```python
from build123d import *

# Parameters (mm, degrees)
SKETCH1_W           = 2.5
SKETCH1_H           = 2.5
SKETCH1_W_2         = 2
SKETCH1_H_2         = 2
BOSS_EXTRUDE1_DEPTH = 2.5
SCALE1_SCALE        = 6


with BuildPart() as part:
    # Sketch1 → Boss-Extrude1 (new body)
    with BuildSketch(Plane(origin=(0, 0, 0), x_dir=(1, 0, 0), z_dir=(0, 1, 0))):
        Rectangle(SKETCH1_W, SKETCH1_H)
        Rectangle(SKETCH1_W_2, SKETCH1_H_2, mode=Mode.SUBTRACT)
    extrude(amount=BOSS_EXTRUDE1_DEPTH)


with BuildPart() as part_1:
    # Scale1: scaled about (0, 1.25, 0)
    add(part.part.scale(SCALE1_SCALE).moved(Location((0, -6.25, 0))))


solid = part_1.part
```
Verification items for the finished model (mm, model axes). A direction names the side the tool comes from. Coordinates: 2 decimals unless noted, no trailing zeros. Loops run counter-clockwise (first coordinate to the right, second up) from the corner with the lowest first, then second, coordinate; pieces in that order, holes last. Notation, with made-up numbers: (-30, 81.5) -> (12, 81.5) arc R16 ccw to (12, 109.5) -> close; hole circle Ø7 at (-16, -28). An arc over 180 degrees is marked (long way). Put each result on its own line as item: value.
1. Section check C-C, the plane y = 7.75. Record the boundary of the cut face in (x, z).
Result set:
outline: (-7.5, -7.5) -> (7.5, -7.5) -> (7.5, 7.5) -> (-7.5, 7.5) -> close; hole (-6, -6) -> (6, -6) -> (6, 6) -> (-6, 6) -> close
2. Section check B-B, the plane z = -3.25. Record the boundary of the cut face in (x, y), then the cut area to 3 significant figures.
Result set:
outline: (-7.5, -6.25) -> (-6, -6.25) -> (-6, 8.75) -> (-7.5, 8.75) -> close; (6, -6.25) -> (7.5, -6.25) -> (7.5, 8.75) -> (6, 8.75) -> close
area: 45.0 mm^2
3. Tool access check on faces 1 (the face through (0, 1, 6)), 2 (the face through (0, 1, -7.5)). Record the directions out of +Z, -Z, +X, -X, +Y, -Y that give a thin tool (end or side, any length) a straight path to the whole face; none if there is none.
Result set:
face 1: +Y, -Y
face 2: -Z, +X, -X, +Y, -Y
4. Mould release check, pull along Z, two halves, no side actions. Record for faces 3 (the face through (0, 1, 7.5)), 4 (the face through (0, 1, -6)), 5 (the face through (6, 1, 0)), 6 (the face through (7.5, 1, 0)): pulls with the +Z half, pulls with the -Z half, needs draft (parallel to the pull), parting line crosses it, or undercut.
Result set:
face 3: pulls with the +Z half
face 4: undercut
face 5: undercut
face 6: needs draft
5. Thickness scan on line 1 (Z direction, x = 5, y = -2.25). Record the ranges inside material, lowest first.
Result set:
line 1: z = -7.5 to -6, 6 to 7.5
6. Section check A-A, the plane x = -4.25. Record the boundary of the cut face in (y, z), then the cut area to 3 significant figures.
Result set:
outline: (-6.25, -7.5) -> (8.75, -7.5) -> (8.75, -6) -> (-6.25, -6) -> close; (-6.25, 6) -> (8.75, 6) -> (8.75, 7.5) -> (-6.25, 7.5) -> close
area: 45.0 mm^2
